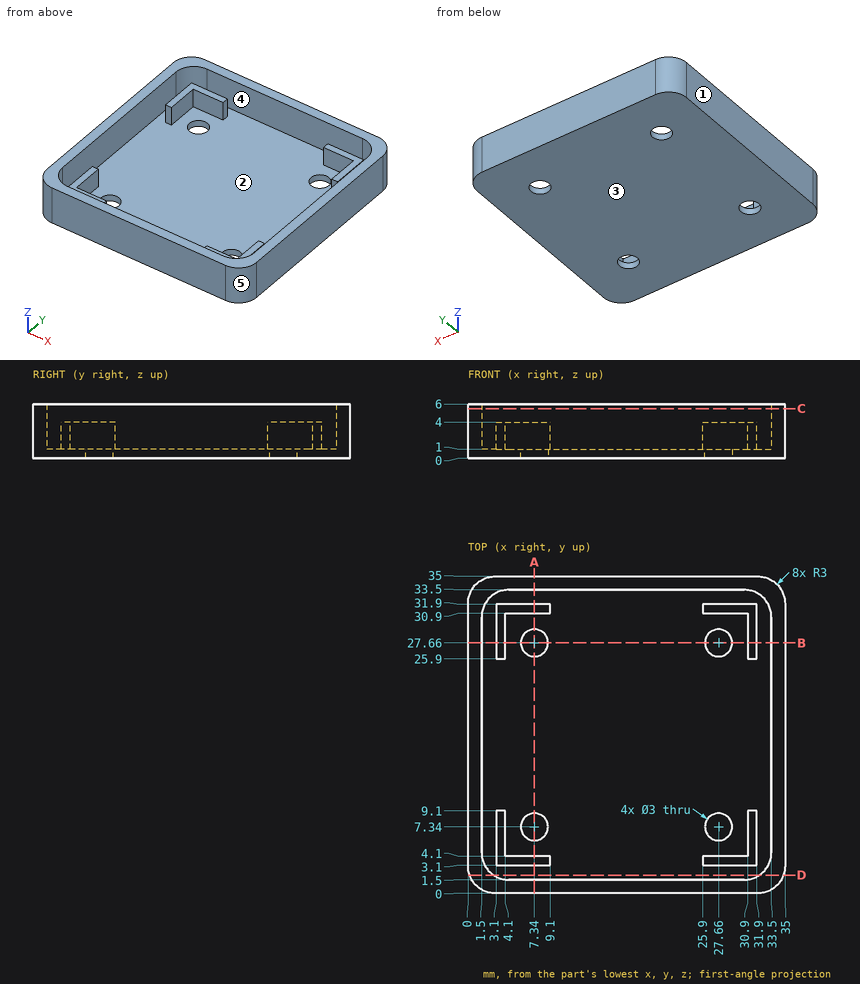
Could you check a few things on this drawing? It's one solid part, dimensions in mm from its lowest x, y, z. A direction names the side the tool comes from. Round coordinates to 2 decimals unless told otherwise and drop trailing zeros. Order: outer loops, then holes, each group sorted by start corner. A loop starts at its lowest first (then second) coordinate and runs counter-clockwise, first axis right, second up.
(1) If we mould it in two halves opening along X, with no side actions, what happens to the marked faces 1, 2 and 3? For each: released by +X, released by -X, zero draft, split by the parting line, or undercut.
Response values:
face 1: released by -X
face 2: undercut
face 3: zero draft
(2) Imagine slicing it at C-C (z = 5.5). Write out the boundary of the cut face in (x, y).
Response values:
outline: (0, 3) arc R3 ccw to (3, 0) - (32, 0) arc R3 ccw to (35, 3) - (35, 32) arc R3 ccw to (32, 35) - (3, 35) arc R3 ccw to (0, 32) - close; hole (1.5, 4.5) arc R3 ccw to (4.5, 1.5) - (30.5, 1.5) arc R3 ccw to (33.5, 4.5) - (33.5, 30.5) arc R3 ccw to (30.5, 33.5) - (4.5, 33.5) arc R3 ccw to (1.5, 30.5) - close
(3) Imagine slicing it at A-A (x = 7.34). Write out the boundary of the cut face in (y, z).
Response values:
outline: (0, 0) - (5.84, 0) - (5.84, 1) - (4.1, 1) - (4.1, 4) - (3.1, 4) - (3.1, 1) - (1.5, 1) - (1.5, 6) - (0, 6) - close; (8.84, 0) - (26.16, 0) - (26.16, 1) - (8.84, 1) - close; (29.16, 0) - (35, 0) - (35, 6) - (33.5, 6) - (33.5, 1) - (31.9, 1) - (31.9, 4) - (30.9, 4) - (30.9, 1) - (29.16, 1) - close
(4) Imagine slicing it at D-D (y = 2). Write out the boundary of the cut face in (x, z), plus the area to 3 significant figures.
Response values:
outline: (0.17, 0) - (34.83, 0) - (34.83, 6) - (32.16, 6) - (32.16, 1) - (2.84, 1) - (2.84, 6) - (0.17, 6) - close
area: 61.4 mm2
(5) Please list where these lines run through material, in increasing order: line 1 along Y through (x, z) = (27.66, 0.35); line 2 along Y through (x, z) = (9, 3.65); line 3 along Y through (x, z) = (15.5, 2.3).
Response values:
line 1: y = 0 to 5.84, 8.84 to 26.16, 29.16 to 35
line 2: y = 0 to 1.5, 3.1 to 4.1, 30.9 to 31.9, 33.5 to 35
line 3: y = 0 to 1.5, 33.5 to 35
(6) Which directions (+Z, -Z, +X, -X, +Y, -Y) give clear straight access to the entire face, cutting with the end or side of a thin tool? Please do the marked faces 4 and 5.
Response values:
face 4: +Z
face 5: +Z, -Z, +X, -Y
(7) I'm going to push flat-ended pins straight in: pin 1 (3 mm diameter, centred on x = 25, z = 4, fed in from -Y); pin 2 (6.5 mm diameter, centred on x = 5.5, y = 7, fed in from +Z); pin 3 (2.5 mm diameter, centred on x = 27.66, y = 7.34, fed in from +Z). Where does each tip first touch, or does it pass through?
Response values:
pin 1: stops at y = 0
pin 2: stops at z = 4
pin 3: passes through
